Source: three-view drawing plus pictorial views. Frame: mm from the lowest corner of the part. A direction names the side the tool comes from. Coordinates: 2 decimals unless noted, no trailing zeros. Write each loop counter-clockwise with the first axis right and the second up, starting at its lowest first coordinate (ties: lowest second). Pieces come first, ordered by that corner, then holes. Notation, with made-up numbers: (-9, 34.5) - (-3, 34.5) arc R3 cw to (-3, 39.5) - close; hole circle Ø2 at (25.5, 53.5). An arc over 180 degrees is marked (long way). Put each result on its own line as item: value.
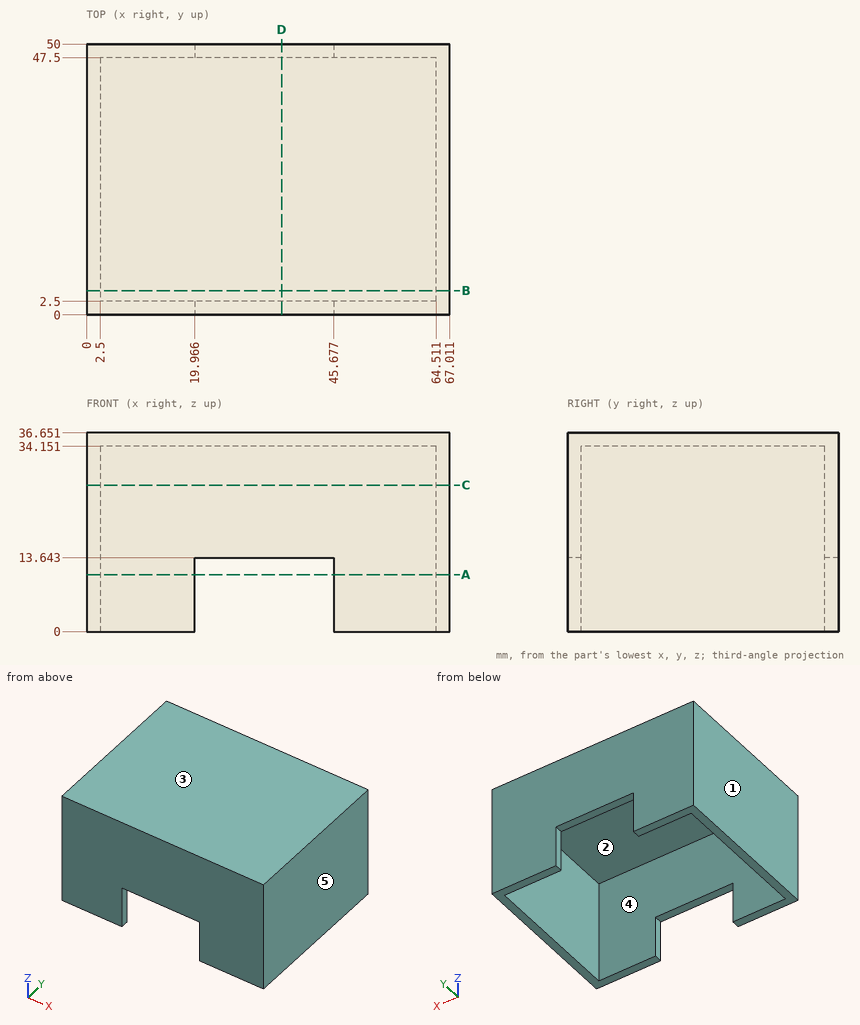
1. Set-up query: the marked faces 4 and 5. Return all of +Z, -Z, +X, -X, +Y, -Y with unobstructed straight access to the full face (end or side cutting, diameter ignored); none if empty.
Answer below:
face 4: -Z
face 5: +Z, -Z, +X, +Y, -Y
2. Section query C-C (z = 27). Return loops of the section in (x, y).
Answer below:
outline: (0, 0) - (67.01, 0) - (67.01, 50) - (0, 50) - close; hole (2.5, 2.5) - (64.51, 2.5) - (64.51, 47.5) - (2.5, 47.5) - close
3. Section query A-A (z = 10.5). Return loops of the section in (x, y).
Answer below:
outline: (0, 0) - (19.97, 0) - (19.97, 2.5) - (2.5, 2.5) - (2.5, 47.5) - (19.97, 47.5) - (19.97, 50) - (0, 50) - close; (45.68, 0) - (67.01, 0) - (67.01, 50) - (45.68, 50) - (45.68, 47.5) - (64.51, 47.5) - (64.51, 2.5) - (45.68, 2.5) - close
4. Mould query, pull axis Z, two halves, no side actions, for the marked faces 1, 2 and 3. Classes: +Z half, -Z half, draft (parallel to the pull), parting line (faces both ways), or undercut.
Answer below:
face 1: draft
face 2: -Z half
face 3: +Z half
5. Pin query (flat end, axial travel): pin 1 Ø1.2 at (x, y) = (29.5, 48.5) entering from -Z; pin 2 Ø13.5 at (x, y) = (44, 31) entering from -Z. Return the tip coordinate at first contact, or that it passes through.
Answer below:
pin 1: stops at z = 13.64
pin 2: stops at z = 34.15
6. Section query B-B (y = 4.5). Return loops of the section in (x, z).
Answer below:
outline: (0, 0) - (2.5, 0) - (2.5, 34.15) - (64.51, 34.15) - (64.51, 0) - (67.01, 0) - (67.01, 36.65) - (0, 36.65) - close
7. Ray query, probe 1 along X at (y, z) = (32.5, 23.5); probe 2 along Y at (x, z) = (52, 2.5); probe 3 along Z at (x, y) = (12.5, 20). Return the intervals inside material, ascending. Write a range as from..to.
Answer below:
probe 1: x = 0..2.5, 64.51..67.01
probe 2: y = 0..2.5, 47.5..50
probe 3: z = 34.15..36.65
8. Section query D-D (x = 36). Return loops of the section in (y, z).
Answer below:
outline: (0, 13.64) - (2.5, 13.64) - (2.5, 34.15) - (47.5, 34.15) - (47.5, 13.64) - (50, 13.64) - (50, 36.65) - (0, 36.65) - close
